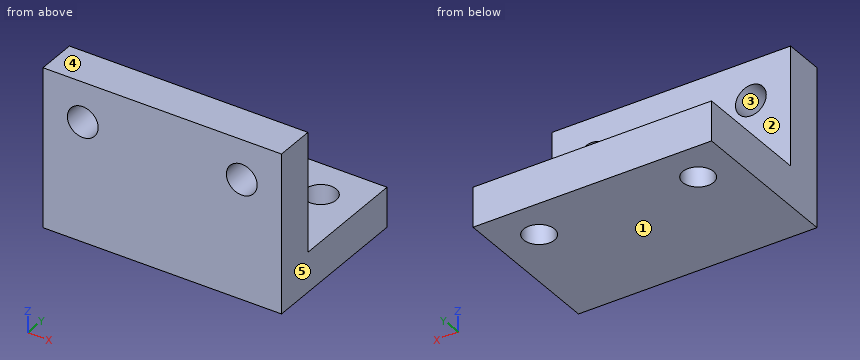
from build123d import *

# Parameters (mm, degrees)
SKETCH1_W                        = 38.1
SKETCH1_H                        = 25.4
BOSS_EXTRUDE1_DEPTH              = 12.7
CUT_EXTRUDE1_REACH               = 40.1
SKETCH2_W                        = 19.05
SKETCH2_H                        = 19.05
F_10_0_1935_DIAMETER_HOLE2_D     = 4.9149
F_10_0_1935_DIAMETER_HOLE2_DEPTH = 6.35
F_10_0_1935_DIAMETER_HOLE1_D     = 4.9149
F_10_0_1935_DIAMETER_HOLE1_DEPTH = 12.7
F_10_0_1935_DIAMETER_HOLE1_TIP   = 1.476584928


with BuildPart() as part:
    # Sketch1 → Boss-Extrude1 (new body, symmetric)
    with BuildSketch(Plane(origin=(0, 0, 0), x_dir=(1, 0, 0), z_dir=(0, 1, 0))):
        Rectangle(SKETCH1_W, SKETCH1_H)
    extrude(amount=BOSS_EXTRUDE1_DEPTH, both=True)

    # Sketch2 → Cut-Extrude1 (cut, up to next)
    with BuildSketch(Plane(origin=(19.05, 0, 0), x_dir=(0, 0, -1), z_dir=(1, 0, 0)), mode=Mode.PRIVATE) as cut_extrude1_sk1:
        with Locations((-3.175, 3.175)):
            Rectangle(SKETCH2_W, SKETCH2_H)
    cut_extrude1_tool1 = extrude(cut_extrude1_sk1.sketch, amount=-CUT_EXTRUDE1_REACH, mode=Mode.PRIVATE) & part.part
    add(cut_extrude1_tool1.solids().sort_by_distance((19.05, 3.175, 3.175))[0], mode=Mode.SUBTRACT)

    # #10 (0.1935) Diameter Hole2
    with Locations(Plane.XY.offset(-6.35)):
        with Locations((-12.7, 6.35), (12.7, 6.35)):
            Hole(F_10_0_1935_DIAMETER_HOLE2_D / 2, depth=F_10_0_1935_DIAMETER_HOLE2_DEPTH)

    # #10 (0.1935) Diameter Hole1
    with Locations(Plane(origin=(0, -6.35, 0), x_dir=(1, 0, 0), z_dir=(0, 1, 0))):
        with Locations((-12.7, -6.35), (12.7, -6.35)):
            Hole(F_10_0_1935_DIAMETER_HOLE1_D / 2, depth=F_10_0_1935_DIAMETER_HOLE1_DEPTH)
            with Locations((0, 0, -(F_10_0_1935_DIAMETER_HOLE1_DEPTH + F_10_0_1935_DIAMETER_HOLE1_TIP / 2))):  # 118° drill point
                Cone(0, F_10_0_1935_DIAMETER_HOLE1_D / 2, F_10_0_1935_DIAMETER_HOLE1_TIP, mode=Mode.SUBTRACT)


solid = part.part
Geometry: final body of the model. Coordinates: model frame, mm. Face numbers are marked on the shaded views. A direction names the side the tool comes from. Give positions to 0.01 mm unless a question says otherwise; leave off trailing zeros. Order: outer loops, then holes, each group sorted by start corner. A loop starts at its lowest first (then second) coordinate and runs counter-clockwise, first axis right, second up. Notation, with made-up numbers: (28, 75) -> (83, 75) arc R10 cw to (83, 86) -> close; hole circle Ø10 at (28.25, 24.25). An arc over 180 degrees is marked (long way). Answer as a JSON object with one key per item and string values.
Q1. Material intervals for probe 1 along Z at (x, y) = (-12.7, -8.75); probe 2 along Y at (x, z) = (-9.5, 2.5), sorted ascending.
Entries:
{"probe 1": "z = -12.7 to 3.89, 8.81 to 12.7", "probe 2": "y = -12.7 to -6.35"}
Q2. Section D-D (x = 4.5). Output: boundary loops of the cut face in (y, z).
Entries:
{"outline": "(-12.7, -12.7) -> (12.7, -12.7) -> (12.7, -6.35) -> (-6.35, -6.35) -> (-6.35, 12.7) -> (-12.7, 12.7) -> close"}
Q3. Section B-B (z = 6.35). Output: boundary loops of the cut face in (x, y).
Entries:
{"outline": "(-19.05, -12.7) -> (-15.16, -12.7) -> (-15.16, -6.35) -> (-19.05, -6.35) -> close; (-10.24, -12.7) -> (10.24, -12.7) -> (10.24, -6.35) -> (-10.24, -6.35) -> close; (15.16, -12.7) -> (19.05, -12.7) -> (19.05, -6.35) -> (15.16, -6.35) -> close"}
Q4. Draft query along X for the marked faces 3, 4 and 5. Return one class per face: released by +X, released by -X, zero draft, split by the parting line, or undercut.
Entries:
{"face 3": "undercut", "face 4": "zero draft", "face 5": "released by +X"}
Q5. First-contact query: pin 1 (6 mm diameter, centred on x = -8, y = 6.5, fed in from +Z); pin 2 (12 mm diameter, centred on x = 13, z = 9, fed in from +Y). Flat tips, straight axial feed; report the tip coordinate or a pass-through.
Entries:
{"pin 1": "stops at z = -6.35", "pin 2": "stops at y = -6.35"}
Q6. Access query for the marked faces 1 and 2. Directions: +Z, -Z, +X, -X, +Y, -Y. A direction counts if a zero-diameter tool reaches every point of the face in a straight line with its end or side. Return the directions, or none.
Entries:
{"face 1": "-Z, +X, -X, +Y, -Y", "face 2": "+Z, +X, -X, +Y"}
Q7. Section A-A (x = 12.7). Output: boundary loops of the cut face in (y, z), plus the area to 3 significant figures.
Entries:
{"outline": "(-12.7, -12.7) -> (3.89, -12.7) -> (3.89, -6.35) -> (-6.35, -6.35) -> (-6.35, 3.89) -> (-12.7, 3.89) -> close; (-12.7, 8.81) -> (-6.35, 8.81) -> (-6.35, 12.7) -> (-12.7, 12.7) -> close; (8.81, -12.7) -> (12.7, -12.7) -> (12.7, -6.35) -> (8.81, -6.35) -> close", "area": "220 mm^2"}
